Print and shaded views of the part. All mm, measured from the part's lowest x, y and z. Give positions to 0.01 mm unless a question says otherwise; leave off trailing zeros. Order: outer loops, then holes, each group sorted by start corner. A loop starts at its lowest first (then second) coordinate and runs counter-clockwise, first axis right, second up. Notation, with made-up numbers: (39.5, 8) - (96.5, 8) arc R23 cw to (96.5, 26) - close; hole circle Ø6 at (25, 65). An arc over 180 degrees is marked (long way). Answer in a Markdown table with one row per item.
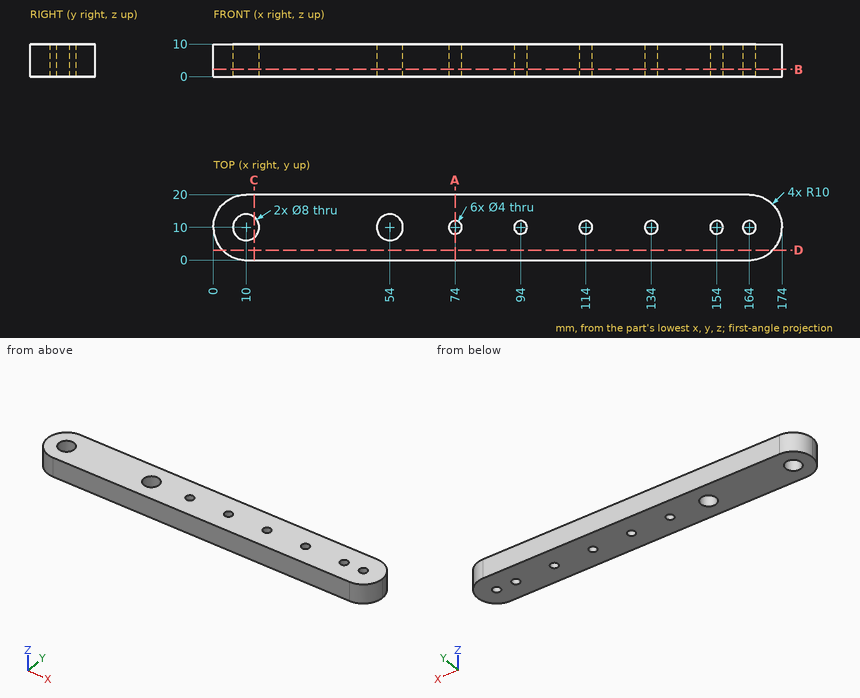
1. Probe line 1 (Y direction, x = 74, z = 6); line 2 (Y direction, x = 54, z = 7.75); line 3 (X direction, y = 12.75, z = 8.5) (1 decimal). List the from-to ranges inside material, lowest first.
Check result:
| item | result |
|---|---|
| line 1 | y = 0 to 8, 12 to 20 |
| line 2 | y = 0 to 6, 14 to 20 |
| line 3 | x = 0.4 to 7.1, 12.9 to 51.1, 56.9 to 173.6 |
2. Drop flat-ended pins along their axis: P1, Ø4, axis at y = 3.5, z = 6, coming from the -X side; P2, Ø4, axis at y = 14.5, z = 3.5, coming from the +X side; P3, Ø6.5, axis at x = 10, y = 10, coming from the +Z side; P4, Ø3, axis at y = 4.5, z = 5, coming from the +X side (3 decimals). Give the stop position or say it passes through.
Check result:
| item | result |
|---|---|
| P1 | stops at x = 1.07 |
| P2 | stops at x = 173.68 |
| P3 | passes through |
| P4 | stops at x = 173.165 |
3. Cut at B-B on z = 2.25. Count the separate pieces of the cut face and the enclosed holes in it, and give its area (3 significant figures).
Check result:
| item | result |
|---|---|
| separate pieces | 1 |
| enclosed holes | 8 |
| area | 3,220 mm² |
4. Cut at D-D on y = 3. Write the cut outline in (x, z).
Check result:
| item | result |
|---|---|
| outline | (2.86, 0) - (171.14, 0) - (171.14, 10) - (2.86, 10) - close |
5. Cut at A-A on x = 74. Write the cut outline in (y, z).
Check result:
| item | result |
|---|---|
| outline | (0, 0) - (8, 0) - (8, 10) - (0, 10) - close; (12, 0) - (20, 0) - (20, 10) - (12, 10) - close |
6. Cut at C-C on x = 12.5. Write the cut outline in (y, z).
Check result:
| item | result |
|---|---|
| outline | (0, 0) - (6.88, 0) - (6.88, 10) - (0, 10) - close; (13.12, 0) - (20, 0) - (20, 10) - (13.12, 10) - close |
